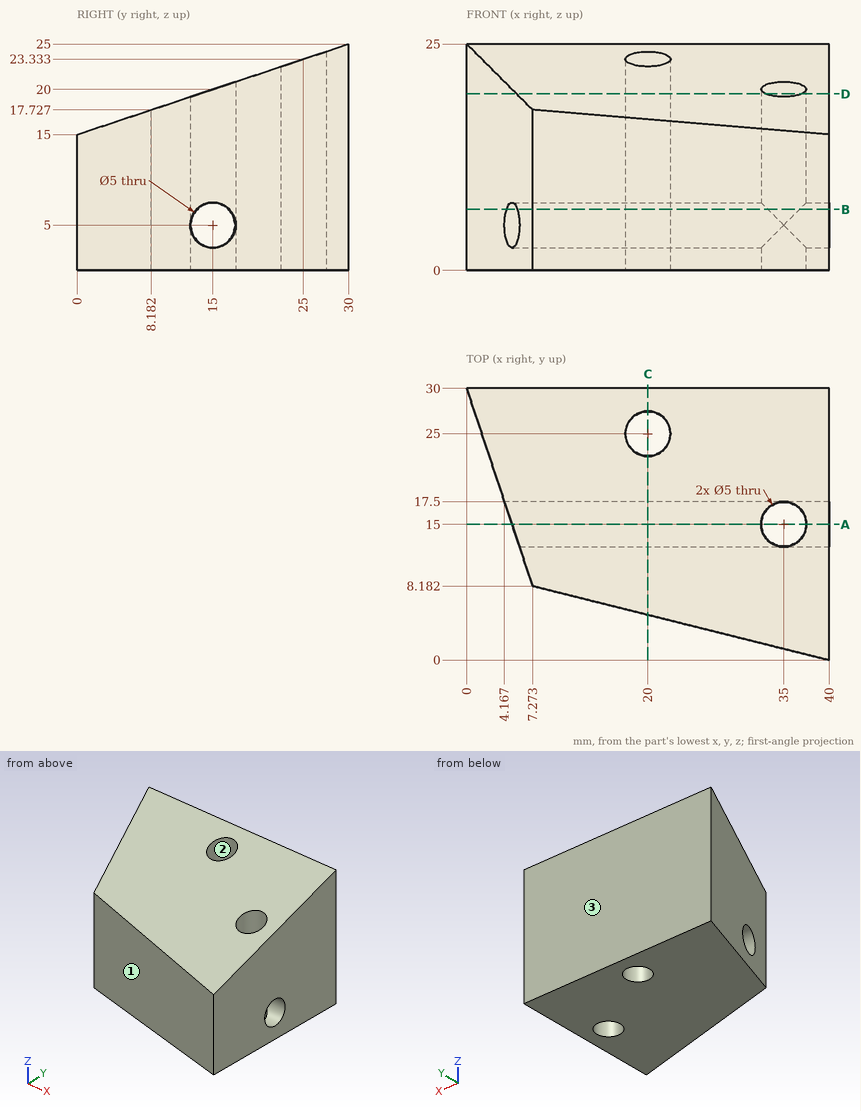
Can you work these out from the drawing? Everything is in mm from the part's minimum corner. Round coordinates to 2 decimals unless told otherwise and drop trailing zeros. Loops run counter-clockwise (first coordinate to the right, second up) from the corner with the lowest first, then second, coordinate; pieces in that order, holes last. Notation, with made-up numbers: (40, 14) -> (94, 14) arc R23 cw to (94, 25) -> close; hole circle Ø10 at (3, 49.5). An arc over 180 degrees is marked (long way). Answer in a Markdown table with one row per item.
Item 1: Suppose I cut it at B-B, the plane z = 6.75. Give the number of separate pieces and of enclosed holes in the cut face, plus the area to 3 significant figures.
Answer block:
| item | result |
|---|---|
| separate pieces | 2 |
| enclosed holes | 1 |
| area | 779 mm² |
Item 2: Suppose I cut it at C-C, the plane x = 20. List the corners of the cut face in (y, z) for me.
Answer block:
| item | result |
|---|---|
| outline | (5, 0) -> (22.5, 0) -> (22.5, 22.5) -> (5, 16.67) -> close; (27.5, 0) -> (30, 0) -> (30, 25) -> (27.5, 24.17) -> close; hole circle Ø5 at (15, 5) |
Item 3: Suppose I cut it at A-A, the plane y = 15. List the corners of the cut face in (x, z) for me.
Answer block:
| item | result |
|---|---|
| outline | (5, 0) -> (32.5, 0) -> (32.5, 2.5) -> (5, 2.5) -> close; (5, 7.5) -> (32.5, 7.5) -> (32.5, 20) -> (5, 20) -> close; (37.5, 0) -> (40, 0) -> (40, 2.5) -> (37.5, 2.5) -> close; (37.5, 7.5) -> (40, 7.5) -> (40, 20) -> (37.5, 20) -> close |
Item 4: Will these pins go through, and if not, where does the flat tip stop? P1, Ø6, axis at x = 20, y = 25, coming from the +Z side; P2, Ø6, axis at x = 11.5, y = 3.5, coming from the +Z side; P3, Ø5, axis at x = 16, z = 11, coming from the -Y side (1 decimal); P4, Ø10, axis at y = 19.5, z = 10, coming from the -X side.
Answer block:
| item | result |
|---|---|
| P1 | z = 24.33 |
| P2 | through |
| P3 | y = 5.4 |
| P4 | x = 1.83 |
Item 5: We'd pull the mould along Y, two halves only. Please class the marked faces 1, 2 and 3: released by +Y, released by -Y, zero draft, split by the parting line, or undercut.
Answer block:
| item | result |
|---|---|
| face 1 | released by -Y |
| face 2 | undercut |
| face 3 | released by +Y |
Item 6: If I drill on probe 1 along X at (y, z) = (15, 10); probe 2 along Y at (x, z) = (20, 16.25); probe 3 along X at (y, z) = (25, 10.5), over which ranges is the centre line in solid material (lowest first)?
Answer block:
| item | result |
|---|---|
| probe 1 | 5 to 32.5, 37.5 to 40 |
| probe 2 | 5 to 22.5, 27.5 to 30 |
| probe 3 | 1.67 to 17.5, 22.5 to 40 |
Item 7: Suppose I cut it at D-D, the plane z = 19.5. List the corners of the cut face in (x, y) for me, plus the area to 3 significant figures.
Answer block:
| item | result |
|---|---|
| outline | (0, 30) -> (5.5, 13.5) -> (33, 13.5) arc R2.5 cw (long way) to (37, 13.5) -> (40, 13.5) -> (40, 30) -> close; hole circle Ø5 at (20, 25) |
| area | 578 mm² |
